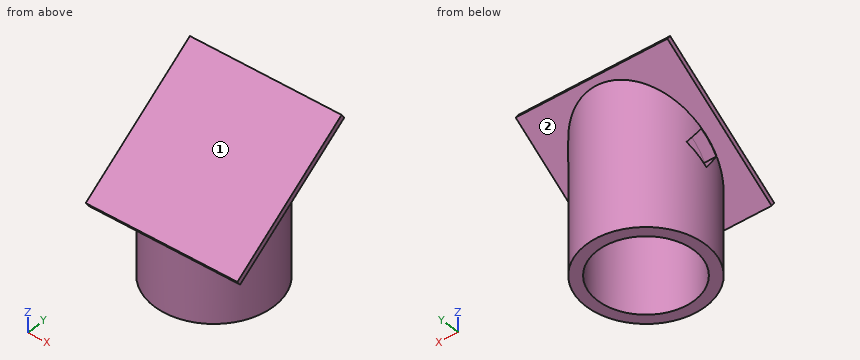
from build123d import *

# Parameters (mm, degrees)
BOX059_W               = 30
BOX059_H               = 13
BOX059_DEPTH           = 13
BOX059_PLACEMENT_ANGLE = 55
BOX057_W               = 90
BOX057_H               = 40
BOX057_DEPTH           = 90
BOX057_PLACEMENT_ANGLE = 55
CYLINDER032_R          = 25.5
CYLINDER032_DEPTH      = 80
CYLINDER033_R          = 31.5
CYLINDER033_DEPTH      = 80
BOX058_W               = 80
BOX058_H               = 80.5
BOX058_DEPTH           = 3
BOX058_ROLL_ANGLE      = 35


with BuildPart() as usb_hole:
    # Box059 → Box059 (new body)
    with BuildSketch(Plane.XY):
        with Locations((15, 6.5)):
            Rectangle(BOX059_W, BOX059_H)
    extrude(amount=BOX059_DEPTH)


with BuildPart() as usb_hole_1:
    # Box059 placement: moved
    add(usb_hole.part.moved(Location((3, 51, 16))).rotate(Axis((3, 51, 16), (-1, 0, 0)), BOX059_PLACEMENT_ANGLE))


with BuildPart() as cube012:
    # Box057 → Box057 (new body)
    with BuildSketch(Plane.XY):
        with Locations((45, 20)):
            Rectangle(BOX057_W, BOX057_H)
    extrude(amount=BOX057_DEPTH)


with BuildPart() as cube012_1:
    # Box057 placement: moved
    add(cube012.part.moved(Location((0, -12, 68))).rotate(Axis((0, -12, 68), (-1, 0, 0)), BOX057_PLACEMENT_ANGLE))


with BuildPart() as cylinder017:
    # Cylinder032 → Cylinder032 (new body)
    with BuildSketch(Plane(origin=(41, 43, 0), x_dir=(1, 0, 0), z_dir=(0, 0, 1))):
        Circle(CYLINDER032_R)
    extrude(amount=CYLINDER032_DEPTH)


with BuildPart() as cut061:
    # Cylinder033 → Cylinder033 (new body)
    with BuildSketch(Plane(origin=(41, 43, 0), x_dir=(1, 0, 0), z_dir=(0, 0, 1))):
        Circle(CYLINDER033_R)
    extrude(amount=CYLINDER033_DEPTH)

    # Cut060: cut Cylinder017
    add(cylinder017.part, mode=Mode.SUBTRACT)

    # Cut061: cut Cube012
    add(cube012_1.part, mode=Mode.SUBTRACT)


with BuildPart() as cut061_1:
    # Cut061 placement: moved
    add(cut061.part.moved(Location((0, 16, -35))))


with BuildPart() as tube_to_tablet_piece:
    # Box058 → Box058 (new body)
    with BuildSketch(Plane.XY):
        with Locations((40, 40.25)):
            Rectangle(BOX058_W, BOX058_H)
    extrude(amount=BOX058_DEPTH)


with BuildPart() as tube_to_tablet_piece_1:
    # Box058 roll: moved
    add(tube_to_tablet_piece.part.rotate(Axis((0, 0, 0), (1, 0, 0)), BOX058_ROLL_ANGLE))


with BuildPart() as tube_to_tablet_piece_2:
    # Box058 placement: moved
    add(tube_to_tablet_piece_1.part.moved(Location((1, 27.5, 0))))

    # Fusion101: union Cut061
    add(cut061_1.part)

    # Cut062: cut USB hole
    add(usb_hole_1.part, mode=Mode.SUBTRACT)


with BuildPart() as tube_to_tablet_piece_3:
    # Cut062 placement: moved
    add(tube_to_tablet_piece_2.part.moved(Location((-37, 74, 1348))))


solid = tube_to_tablet_piece_3.part
Could you check a few things on this model? Use its own coordinates, in mm. Face numbers are marked on the shaded views. Give positions to 0.01 mm unless a question says otherwise; leave off trailing zeros. Order: outer loops, then holes, each group sorted by start corner. A loop starts at its lowest first (then second) coordinate and runs counter-clockwise, first axis right, second up.
1. Suppose I cut it at D-D (z = 1375). List the corners of the cut face in (x, y) for me.
2. I need wall thicknesses on L1, parallel to X at y = 133, z = 1352; L2, parallel to Y at x = 4, z = 1338; L3, parallel to X at y = 133, z = 1362. Which ranges of each line are inside material? Lowest first, please.
3. Will these pins go through, and if not, where does the flat tip stop? P1, Ø5, axis at y = 137, z = 1326, coming from the -X side; P2, Ø10, axis at x = 34, z = 1382, coming from the +Y side; P3, Ø8, axis at y = 116, z = 1353.5, coming from the +X side; P4, Ø10, axis at x = -21.5, z = 1358.5, coming from the +Y side.
4. We'd pull the mould along Y, two halves only. Please class the marked faces 1 and 2: pulls with the +Y half, pulls with the -Y half, needs draft (parallel to the pull), parting line crosses it, or undercut.
5. Suppose I cut it at B-B (x = -18). List the corners of the cut face in (y, z) for me.
6. Suppose I cut it at A-A (y = 129). List the corners of the cut face in (x, z) for me (3 decimals).
Solved:
1. outline: (-36, 134.83) - (44, 134.83) - (44, 140.06) - (34.7, 140.06) arc R31.5 ccw to (-26.7, 140.06) - (-36, 140.06) - close; hole (-20.5, 140.06) - (28.5, 140.06) arc R25.5 ccw to start
2. L1: x = -27.5 to -21.5, 29.5 to 35.5
2. L2: y = 101.5 to 107.5, 158.5 to 164.5
2. L3: x = 29.5 to 35.5
3. P1: stops at x = -27.46
3. P2: stops at y = 157.2
3. P3: stops at x = 44
3. P4: stops at y = 156.92
4. face 1: pulls with the -Y half
4. face 2: undercut
5. outline: (99.78, 1350.46) - (101.5, 1348) - (110.46, 1354.27) - (110.46, 1313) - (120.11, 1313) - (120.11, 1361.03) - (145.89, 1379.08) - (145.89, 1313) - (155.54, 1313) - (155.54, 1385.84) - (167.44, 1394.17) - (165.72, 1396.63) - close
6. outline: (-36, 1367.256) - (-27.245, 1367.256) - (-27.245, 1366.801) - (-21.184, 1366.801) - (-21.184, 1367.256) - (29.184, 1367.256) - (29.184, 1313) - (35.245, 1313) - (35.245, 1367.256) - (44, 1367.256) - (44, 1370.918) - (-36, 1370.918) - close; (-27.245, 1313) - (-21.184, 1313) - (-21.184, 1358.287) - (-27.245, 1358.287) - close
